```python
from build123d import *

# Parameters (mm, degrees)
F1_DEPTH = 2


with BuildPart() as f1:
    # F0 (on Top) → F1 (new body)
    with BuildSketch(Plane.XY):
        Polygon((27.954835, -79.590207), (23.561089, 96.622099), (-23.264273, 96.622099), (-27.658019, -79.590207), align=None)
        with BuildLine():
            Line((-21.592149, -60.128083), (-19.099485, 39.840846))
            ThreePointArc((-19.099485, 39.840846), (-16.537945, 42.277752), (-14.101039, 39.716212))
            Line((-14.101039, 39.716212), (-16.593702, -60.252716))
            ThreePointArc((-16.593702, -60.252716), (-19.155242, -62.689622), (-21.592149, -60.128083))
        make_face(mode=Mode.SUBTRACT)
        with BuildLine():
            ThreePointArc((14.397855, 39.716212), (16.834762, 42.277752), (19.396301, 39.840846))
            Line((19.396301, 39.840846), (21.888965, -60.128083))
            ThreePointArc((21.888965, -60.128083), (19.452058, -62.689622), (16.890518, -60.252716))
            Line((16.890518, -60.252716), (14.397855, 39.716212))
        make_face(mode=Mode.SUBTRACT)
    extrude(amount=F1_DEPTH)


solid = f1.part
```
Check sheet for the modelled part. Datum: model origin and axes. Units: mm. Round coordinates to 2 decimals unless told otherwise and drop trailing zeros. Loops run counter-clockwise (first coordinate to the right, second up) from the corner with the lowest first, then second, coordinate; pieces in that order, holes last. Notation, with made-up numbers: M -7.5,-12.75 L -1.5,-12.75 A24 ccw -1.5,11.25 Z; hole C 29.5,77 d6. An arc over 180 degrees is marked long. Answer as a JSON object with one key per item and string values.
1. Section check C-C (y = 17.5). Record the boundary of the cut face in (x, z), plus the area to 3 significant figures.
Reply:
{"outline": "M -25.24,0 L -19.66,0 L -19.66,2 L -25.24,2 Z; M -14.65,0 L 14.95,0 L 14.95,2 L -14.65,2 Z; M 19.95,0 L 25.53,0 L 25.53,2 L 19.95,2 Z", "area": "81.5 mm²"}
2. Section check B-B (y = -15). Record the boundary of the cut face in (x, z), plus the area to 3 significant figures.
Reply:
{"outline": "M -26.05,0 L -20.47,0 L -20.47,2 L -26.05,2 Z; M -15.47,0 L 15.76,0 L 15.76,2 L -15.47,2 Z; M 20.76,0 L 26.34,0 L 26.34,2 L 20.76,2 Z", "area": "84.8 mm²"}
3. Section check A-A (z = 0.55). Record the boundary of the cut face in (x, y), plus the area to 3 significant figures.
Reply:
{"outline": "M -27.66,-79.59 L 27.95,-79.59 L 23.56,96.62 L -23.26,96.62 Z; hole M -21.59,-60.13 A2.5 ccw -16.59,-60.25 L -14.1,39.72 A2.5 ccw -19.1,39.84 Z; hole M 14.4,39.72 L 16.89,-60.25 A2.5 ccw 21.89,-60.13 L 19.4,39.84 A2.5 ccw Z", "area": "7,990 mm²"}
4. Scan lines: line 1 (X direction, y = 27, z = 1.85); line 2 (X direction, y = 24.5, z = 0.85); line 3 (X direction, y = 43.5, z = 0.45). Record each from-to range of solid material in increasing order.
Reply:
{"line 1": "x = -25 to -19.42, -14.42 to 14.71, 19.72 to 25.3", "line 2": "x = -25.06 to -19.48, -14.48 to 14.78, 19.78 to 25.36", "line 3": "x = -24.59 to 24.89"}
